Design review of the part built by this model. Coordinates are the model's own, in mm. A direction names the side the tool comes from. Coordinates: 2 decimals unless noted, no trailing zeros. Loops run counter-clockwise (first coordinate to the right, second up) from the corner with the lowest first, then second, coordinate; pieces in that order, holes last. Notation, with made-up numbers: (14, 45.5) -> (65, 45.5) arc R17 cw to (65, 67.5) -> close; hole circle Ø6 at (82.25, -39.5). An arc over 180 degrees is marked (long way). Answer in a Markdown table with one row per item.
```python
from build123d import *

# Parameters (mm, degrees)
SZKIC1_W                    = 95.25
SZKIC1_H                    = 50.8
SZKIC1_R                    = 1.83
DODANIE_WYCI_GNI_CIE1_DEPTH = 2.54
SZKIC2_W                    = 76.2
SZKIC2_H                    = 50.8
DODANIE_WYCI_GNI_CIE2_DEPTH = 20.32
OTW_R_50_0_07_1_D           = 1.778
OTW_R_50_0_07_1_DEPTH       = 5
OTW_R_50_0_07_1_TIP         = 0.53416509
SZKIC6_R                    = 3.5
DODANIE_WYCI_GNI_CIE3_DEPTH = 11
SZKIC7_R                    = 5
DODANIE_WYCI_GNI_CIE4_DEPTH = 1
DODANIE_WYCI_GNI_CIE5_START = 11
SZKIC8_R                    = 3.5
DODANIE_WYCI_GNI_CIE5_DEPTH = 11
DODANIE_WYCI_GNI_CIE6_START = 1
SZKIC9_R                    = 5
DODANIE_WYCI_GNI_CIE6_DEPTH = 1
SZKIC10_R                   = 0.5
DODANIE_WYCI_GNI_CIE7_DEPTH = 10
SZKIC12_R                   = 1.059326458
DODANIE_WYCI_GNI_CIE8_DEPTH = 1
SZKIC11_R                   = 4
DODANIE_WYCI_GNI_CIE9_DEPTH = 1


with BuildPart() as part:
    # Szkic1 → Dodanie-wyciągnięcie1 (new body)
    with BuildSketch(Plane.XY):
        with Locations((-3.430103099, 0.268410085)):
            Rectangle(SZKIC1_W, SZKIC1_H)
        with Locations((-46.060693789, -20.371589915)):
            Circle(SZKIC1_R, mode=Mode.SUBTRACT)
        with Locations((-46.295103099, 20.908410085)):
            Circle(SZKIC1_R, mode=Mode.SUBTRACT)
        with Locations((39.434896901, 20.908410085)):
            Circle(SZKIC1_R, mode=Mode.SUBTRACT)
        with Locations((39.669306211, -20.371589915)):
            Circle(SZKIC1_R, mode=Mode.SUBTRACT)
    extrude(amount=DODANIE_WYCI_GNI_CIE1_DEPTH)

    # Szkic2 → Dodanie-wyciągnięcie2 (add)
    with BuildSketch(Plane.XY.offset(2.54)):
        with Locations((-3.430103099, 0.268410085)):
            Rectangle(SZKIC2_W, SZKIC2_H)
    extrude(amount=DODANIE_WYCI_GNI_CIE2_DEPTH)

    # Otwór #50 (0.07)1
    with Locations(Plane.XY.offset(22.86)):
        with Locations((-37.720103099, 21.858410085), (30.859896901, 21.858410085), (30.859896901, -21.321589915), (-37.720103099, -21.321589915)):
            Hole(OTW_R_50_0_07_1_D / 2, depth=OTW_R_50_0_07_1_DEPTH)
            with Locations((0, 0, -(OTW_R_50_0_07_1_DEPTH + OTW_R_50_0_07_1_TIP / 2))):  # 118° drill point
                Cone(0, OTW_R_50_0_07_1_D / 2, OTW_R_50_0_07_1_TIP, mode=Mode.SUBTRACT)

    # Szkic6 → Dodanie-wyciągnięcie3 (add)
    with BuildSketch(Plane.ZY.offset(41.530103099)):
        with Locations(Location((12.7, -7.351589915, 0), (0, 0, 90))):
            Circle(SZKIC6_R)
    extrude(amount=DODANIE_WYCI_GNI_CIE3_DEPTH)

    # Szkic7 → Dodanie-wyciągnięcie4 (add)
    with BuildSketch(Plane.ZY.offset(41.530103099)):
        with Locations(Location((12.7, -7.351589915, 0), (0, 0, 90))):
            Circle(SZKIC7_R)
    extrude(amount=DODANIE_WYCI_GNI_CIE4_DEPTH)

    # Szkic8 → Dodanie-wyciągnięcie5 (add)
    with BuildSketch(Plane(origin=(34.669896901, 0, 0), x_dir=(0, 0, -1), z_dir=(1, 0, 0)).offset(DODANIE_WYCI_GNI_CIE5_START)):
        with Locations(Location((-12.7, -7.351589915, 0), (0, 0, 270))):
            Circle(SZKIC8_R)
    extrude(amount=-DODANIE_WYCI_GNI_CIE5_DEPTH)

    # Szkic9 → Dodanie-wyciągnięcie6 (add)
    with BuildSketch(Plane(origin=(34.669896901, 0, 0), x_dir=(0, 0, -1), z_dir=(1, 0, 0)).offset(DODANIE_WYCI_GNI_CIE6_START)):
        with Locations(Location((-12.7, -7.351589915, 0), (0, 0, 90))):
            Circle(SZKIC9_R)
    extrude(amount=-DODANIE_WYCI_GNI_CIE6_DEPTH)

    # Szkic10 → Dodanie-wyciągnięcie7 (add)
    with BuildSketch(Plane.ZY.offset(41.530103099)):
        with Locations(Location((10.16, 12.968410085, 0), (0, 0, 90))):
            Circle(SZKIC10_R)
    extrude(amount=DODANIE_WYCI_GNI_CIE7_DEPTH)

    # Szkic12 → Dodanie-wyciągnięcie8 (add)
    with BuildSketch(Plane.ZY.offset(51.530103099)):
        with Locations(Location((10.16, 12.968410085, 0), (0, 0, 270))):
            Circle(SZKIC12_R)
    extrude(amount=-DODANIE_WYCI_GNI_CIE8_DEPTH)

    # Szkic11 → Dodanie-wyciągnięcie9 (add)
    with BuildSketch(Plane.ZY.offset(41.530103099)):
        with Locations(Location((10.16, 12.968410085, 0), (0, 0, 90))):
            Circle(SZKIC11_R)
    extrude(amount=DODANIE_WYCI_GNI_CIE9_DEPTH)


solid = part.part
```
(1) Tool access review of faces 1 (the cylindrical face through (-42.02, -11.32, 15.74)), 2 (the flat face through (39, 1, 2.54)), 3 (the cylindrical face through (40.74, -10.69, 11.65)): name each direction out of +Z, -Z, +X, -X, +Y, -Y from which nothing blocks a thin tool from reaching the whole face with its end or side.
Evaluation:
| item | result |
|---|---|
| face 1 | -X |
| face 2 | +X, +Y, -Y |
| face 3 | +X |
(2) Draft analysis for pull direction X (two halves, no side actions). For faces 4 (the cylindrical face through (-37.065, -20.721, 20.325)), 5 (the flat face through (-41.53, 0, 13)), 6 (the flat face through (35.67, -11, 12)), state which applies: pulls with the +X half, pulls with the -X half, needs draft (parallel to the pull), parting line crosses it, or undercut.
Evaluation:
| item | result |
|---|---|
| face 4 | undercut |
| face 5 | pulls with the -X half |
| face 6 | pulls with the +X half |
(3) Take a section at B-B on z = 21.25. Give the boundary of the cut face in (x, y), and give its area (3 significant figures).
Evaluation:
| item | result |
|---|---|
| outline | (-41.53, -25.13) -> (34.67, -25.13) -> (34.67, 25.67) -> (-41.53, 25.67) -> close; hole circle Ø1.78 at (-37.72, -21.32); hole circle Ø1.78 at (-37.72, 21.86); hole circle Ø1.78 at (30.86, -21.32); hole circle Ø1.78 at (30.86, 21.86) |
| area | 3,860 mm² |
(4) Take a section at A-A on y = 0.5. Give the boundary of the cut face in (x, z).
Evaluation:
| item | result |
|---|---|
| outline | (-51.06, 0) -> (44.19, 0) -> (44.19, 2.54) -> (34.67, 2.54) -> (34.67, 22.86) -> (-41.53, 22.86) -> (-41.53, 2.54) -> (-51.06, 2.54) -> close |
(5) For pin 1 (1.1 mm diameter, centred on y = 13, z = 10.5, fed in from -X); pin 2 (7.5 mm diameter, centred on x = -47.5, y = 0, fed in from +Z); pin 3 (1.6 mm diameter, centred on x = -37.72, y = -21.32, fed in from +Z), all flat-tipped, find the tip position at first contact; note any pin that passes through.
Evaluation:
| item | result |
|---|---|
| pin 1 | stops at x = -51.53 |
| pin 2 | stops at z = 2.54 |
| pin 3 | stops at z = 17.81 |
(6) To check wall thickness, follow probe 1 along X at (y, z) = (-5.5, 16); probe 2 along X at (y, z) = (-12.5, 5); probe 3 along Z at (x, y) = (40, 6). State the ranges of each line that lie inside material, in increasing order.
Evaluation:
| item | result |
|---|---|
| probe 1 | x = -42.53 to 35.67 |
| probe 2 | x = -41.53 to 34.67 |
| probe 3 | z = 0 to 2.54 |
(7) Take a section at C-C on z = 12.7. Give the boundary of the cut face in (x, y).
Evaluation:
| item | result |
|---|---|
| outline | (-52.53, -10.85) -> (-42.53, -10.85) -> (-42.53, -12.35) -> (-41.53, -12.35) -> (-41.53, -25.13) -> (34.67, -25.13) -> (34.67, -12.35) -> (35.67, -12.35) -> (35.67, -10.85) -> (45.67, -10.85) -> (45.67, -3.85) -> (35.67, -3.85) -> (35.67, -2.35) -> (34.67, -2.35) -> (34.67, 25.67) -> (-41.53, 25.67) -> (-41.53, 16.06) -> (-42.53, 16.06) -> (-42.53, 9.88) -> (-41.53, 9.88) -> (-41.53, -2.35) -> (-42.53, -2.35) -> (-42.53, -3.85) -> (-52.53, -3.85) -> close |
